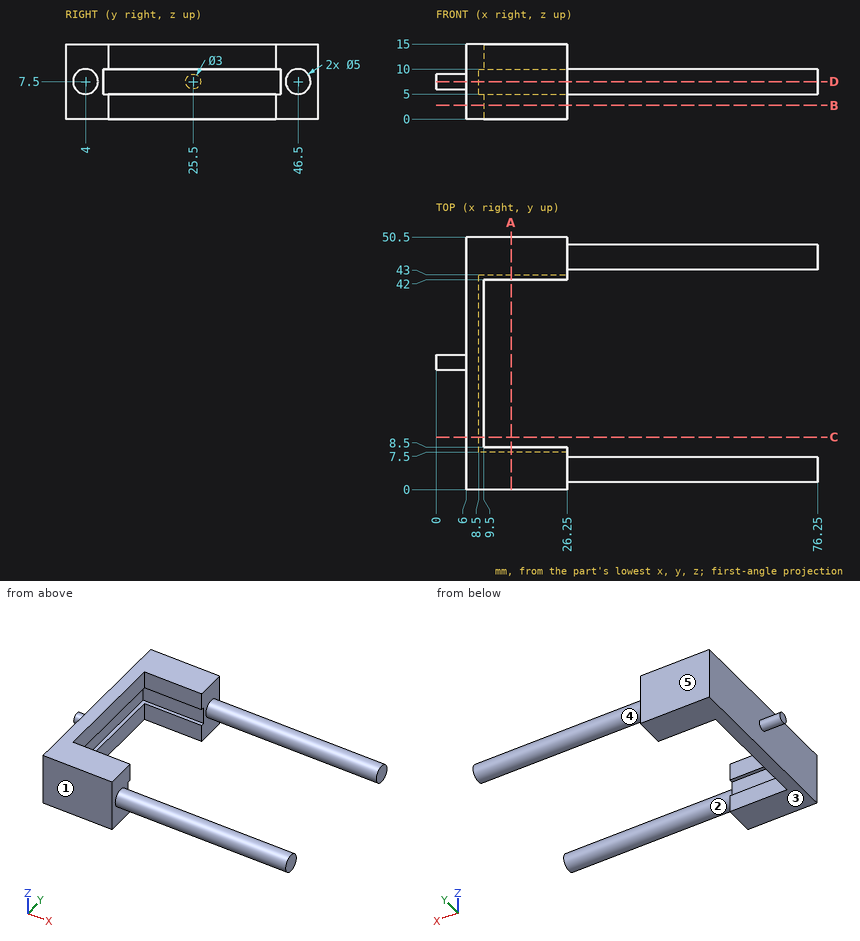
Verification items for this drawing (mm, ordinates from the low corner). A direction names the side the tool comes from. Round coordinates to 2 decimals unless told otherwise and drop trailing zeros. Loops run counter-clockwise (first coordinate to the right, second up) from the corner with the lowest first, then second, coordinate; pieces in that order, holes last. Notation, with made-up numbers: M 76.5,23.25 L 114.5,23.25 A35 ccw 114.5,60.25 Z; hole C -20.75,45.25 d11. An arc over 180 degrees is marked long. Answer as a JSON object with one key per item and string values.
1. Section check C-C (y = 10.5). Record the boundary of the cut face in (x, z).
Reply:
{"outline": "M 6,0 L 9.5,0 L 9.5,5 L 8.5,5 L 8.5,10 L 9.5,10 L 9.5,15 L 6,15 Z"}
2. Mould release check, pull along Y, two halves, no side actions. Record for the marked faces 3, 4 and 5: pulls with the +Y half, pulls with the -Y half, needs draft (parallel to the pull), parting line crosses it, or undercut.
Reply:
{"face 3": "needs draft", "face 4": "undercut", "face 5": "pulls with the +Y half"}
3. Scan lines: line 1 (Y direction, x = 14, z = 12.5); line 2 (X direction, y = 20.5, z = 5.25); line 3 (Z direction, x = 40, y = 48.5). Record each from-to range of solid material in increasing order.
Reply:
{"line 1": "y = 0 to 8.5, 42 to 50.5", "line 2": "x = 6 to 8.5", "line 3": "z = 6 to 9"}
4. Gauge pin test, flat ends, axial feed: P1, Ø8, axis at y = 30.5, z = 13, coming from the -X side; P2, Ø2.5, axis at y = 27.5, z = 13.5, coming from the +X side; P3, Ø5, axis at x = 42, z = 8.5, coming from the -Y side. Record the tip position at first contact, or that the pin passes through.
Reply:
{"P1": "stops at x = 6", "P2": "stops at x = 9.5", "P3": "stops at y = 1.5"}
5. Access from +Z, -Z, +X, -X, +Y, -Y to the whole of each face (thin tool, end or side, straight path). Record for the marked faces 1 and 2.
Reply:
{"face 1": "+Z, -Z, +X, -X, -Y", "face 2": "+X"}
6. Section check A-A (x = 15). Record the boundary of the cut face in (y, z), plus the area to 3 significant figures.
Reply:
{"outline": "M 0,0 L 8.5,0 L 8.5,5 L 7.5,5 L 7.5,10 L 8.5,10 L 8.5,15 L 0,15 Z; M 42,0 L 50.5,0 L 50.5,15 L 42,15 L 42,10 L 43,10 L 43,5 L 42,5 Z", "area": "245 mm²"}
7. Section check B-B (z = 2.75). Record the boundary of the cut face in (x, y), plus the area to 4 significant figures.
Reply:
{"outline": "M 6,0 L 26.25,0 L 26.25,8.5 L 9.5,8.5 L 9.5,42 L 26.25,42 L 26.25,50.5 L 6,50.5 Z", "area": "461.5 mm²"}
8. Section check D-D (z = 7.5). Record the boundary of the cut face in (x, y).
Reply:
{"outline": "M 0,24 L 6,24 L 6,0 L 26.25,0 L 26.25,1.5 L 76.25,1.5 L 76.25,6.5 L 26.25,6.5 L 26.25,7.5 L 8.5,7.5 L 8.5,43 L 26.25,43 L 26.25,44 L 76.25,44 L 76.25,49 L 26.25,49 L 26.25,50.5 L 6,50.5 L 6,27 L 0,27 Z"}
